Verification items for the finished model (mm, model axes). Face numbers are marked on the shaded views. A direction names the side the tool comes from. Round coordinates to 2 decimals unless told otherwise and drop trailing zeros. Order: outer loops, then holes, each group sorted by start corner. A loop starts at its lowest first (then second) coordinate and runs counter-clockwise, first axis right, second up. Notation, with made-up numbers: M -10.75,13.25 L 27.25,13.25 A25 cw 27.25,38.25 Z; hole C -2,26.5 d9. An arc over 180 degrees is marked long. Return JSON: item names as keys, results as strings. Group by question number.
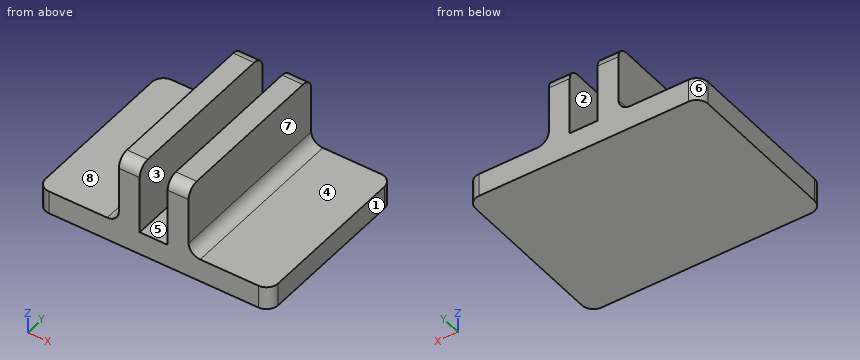
from build123d import *

# Parameters (mm, degrees)
F0_W     = 7
F0_H     = 15
F0_W_2   = 1.8
F0_W_3   = 2.4
F1_DEPTH = 2
F2_DEPTH = 8
F3_R     = 1


with BuildPart() as f1:
    # F0 (on Top) → F1 (new body)
    with BuildSketch(Plane.XY):
        with Locations((-6.5, 0)):
            Rectangle(F0_W, F0_H)
        with Locations((-2.1, 0)):
            Rectangle(F0_W_2, F0_H)
        Rectangle(F0_W_3, F0_H)
        with Locations((2.1, 0)):
            Rectangle(F0_W_2, F0_H)
        with Locations((6.5, 0)):
            Rectangle(F0_W, F0_H)
    extrude(amount=F1_DEPTH)

    # F0 (on Top) → F2 (join)
    with BuildSketch(Plane.XY):
        with Locations((-2.1, 0)):
            Rectangle(F0_W_2, F0_H)
        with Locations((2.1, 0)):
            Rectangle(F0_W_2, F0_H)
    extrude(amount=F2_DEPTH)

    # F3
    f3_edges = [f1.edges().sort_by_distance(p)[0] for p in [
        (2.1, -7.5, 8),
        (-2.1, -7.5, 8),
        (-2.1, 7.5, 8),
        (2.1, 7.5, 8),
        (10, -7.5, 1),
        (10, 7.5, 1),
        (-10, -7.5, 1),
        (-10, 7.5, 1),
        (3, 0, 2),
        (-3, 0, 2),
    ]]
    fillet(f3_edges, radius=F3_R)


solid = f1.part
1. Cross-section at A-A (z = 6.25). Enter the section's corners in (x, y).
2. Cross-section at B-B (y = 2.5). Enter the section's corners in (x, z).
3. Access from +Z, -Z, +X, -X, +Y, -Y to the whole of each face (thin tool, end or side, straight path). Record for the marked faces 5, 6, 7 and 8.
4. Draft check along X on the marked faces 1, 2, 3 and 4. Enter one of: +X half, -X half, draft (parallel to the pull), parting line (faces both ways), or undercut.
5. Thickness scan on line 1 along X through (y, z) = (-6.25, 5.75); line 2 along Z through (x, y) = (-7.75, 5.75); line 3 along X through (y, z) = (-4, 2.25). Record the ranges inside material, lowest first. Write a range as from..to.
6. Cross-section at C-C (x = -8). Enter the section's corners in (y, z).
7. Go/stop test with flat-tipped pins: pin 1 (3 mm diameter, centred on y = -3.5, z = 4, fed in from -X); pin 2 (5 mm diameter, centred on x = 8, y = -2.5, fed in from +Z); pin 3 (1.5 mm diameter, centred on y = 1.5, z = 5.5, fed in from +X). Record where each tip stops, or that it passes through.
8. Cross-section at D-D (x = -3.5). Enter the section's corners in (y, z).
Computed:
{
 "1": {"outline": "M -3,-7.5 L -1.2,-7.5 L -1.2,7.5 L -3,7.5 Z; M 1.2,-7.5 L 3,-7.5 L 3,7.5 L 1.2,7.5 Z"},
 "2": {"outline": "M -10,0 L 10,0 L 10,2 L 4,2 A1 cw 3,3 L 3,8 L 1.2,8 L 1.2,2 L -1.2,2 L -1.2,8 L -3,8 L -3,3 A1 cw -4,2 L -10,2 Z"},
 "3": {"face 5": "+Z, +Y, -Y", "face 6": "+Z, -Z, -X, +Y", "face 7": "+Z, +X, +Y, -Y", "face 8": "+Z, -X, +Y, -Y"},
 "4": {"face 1": "+X half", "face 2": "undercut", "face 3": "undercut", "face 4": "draft"},
 "5": {"line 1": "x = -3..-1.2, 1.2..3", "line 2": "z = 0..2", "line 3": "x = -3.34..-1.2, 1.2..3.34"},
 "6": {"outline": "M -7.5,0 L 7.5,0 L 7.5,2 L -7.5,2 Z"},
 "7": {"pin 1": "stops at x = -3.13", "pin 2": "stops at z = 2", "pin 3": "stops at x = 3"},
 "8": {"outline": "M -7.5,0 L 7.5,0 L 7.5,2.13 L -7.5,2.13 Z"}
}
